Geometry: final body of the model. Coordinates: model frame, mm. Face numbers are marked on the shaded views. A direction names the side the tool comes from. Coordinates: 2 decimals unless noted, no trailing zeros. Order: outer loops, then holes, each group sorted by start corner. A loop starts at its lowest first (then second) coordinate and runs counter-clockwise, first axis right, second up. Notation, with made-up numbers: (-23, 83.5) -> (34, 83.5) arc R21 ccw to (34, 92.5) -> close; hole circle Ø3 at (49, 74.5). An arc over 180 degrees is marked (long way). Answer in a Markdown table with one row per item. Add a question column.
1) Section query B-B on x = -25. Return the cut outline in (y, z).
2) Section query D-D on y = 5. Return the cut outline in (x, z).
3) Section query C-C on y = -3. Return the cut outline in (x, z).
4) Set-up query: the marked faces 4 and 5. Return all of +Z, -Z, +X, -X, +Y, -Y with unobstructed straight access to the full face (end or side cutting, diameter ignored); none if empty.
5) Ray query, line 1 (X direction, y = 4.75, z = 0.2); line 2 (Y direction, x = 0, z = 1.85); line 3 (X direction, y = -14.25, z = 2.5). Return the intervals inside material, ascending. Write a range as from..to.
6) Section query A-A on z = 0.85. Return the cut outline in (x, y), then the cut area to 3 significant figures.
7) Contact query for flat-ended pins moving along their axis: P1, Ø6.5, axis at x = -29.75, y = 5, coming from the -Z side; P2, Ø11, axis at x = -25, y = 3, coming from the +Z side; P3, Ø3.5, axis at x = -15, y = -15.5, coming from the +Z side; P4, Ø2.5, axis at x = 0.25, y = 5, coming from the +Z side. Output: stop coordinate, or through.
8) Pull-direction query (X, two-part tool) for the marked faces 1, 2 and 3; classes: +X half, -X half, draft (parallel to the pull), parting line (faces both ways), or undercut.
```python
from build123d import *

# Parameters (mm, degrees)
EXTRUDE_1_DEPTH     = 2
EXTRUDE_2_DEPTH     = 5
EXTRUDE_3_DEPTH     = 5
SKETCH_4_R          = 2
CUT_EXTRUDE_1_DEPTH = 10
EXTRUDE_START       = -70
EXTRUDE_4_DEPTH     = 70


with BuildPart() as part:
    # 草图1 → 凸台-拉伸1 (new body)
    with BuildSketch(Plane.XY):
        Polygon((-44.754893935, 0), (15.245106065, 0), (15.245106065, -20), (20.245106065, -20), (20.245106065, 10), (15.245106065, 10), (-44.754893935, 10), (-49.754893935, 10), (-49.754893935, -20), (-44.754893935, -20), align=None)
    extrude(amount=EXTRUDE_1_DEPTH)

    # 草图2 → 凸台-拉伸2 (add)
    with BuildSketch(Plane.ZY.offset(49.754893935)):
        Polygon((0, 10), (0, -20), (2, -20), (3.461164558, -13.577882357), (3.461164558, 10), align=None)
    extrude(amount=-EXTRUDE_2_DEPTH)

    # 草图3 → 凸台-拉伸3 (add)
    with BuildSketch(Plane(origin=(20.245106065, 0, 0), x_dir=(0, 0, -1), z_dir=(1, 0, 0))):
        Polygon((-2, 10), (-3.461164558, 10), (-3.461164558, -13.577882357), (-2, -20), align=None)
    extrude(amount=-EXTRUDE_3_DEPTH)

    # 草图4 → 切除-拉伸1 (cut)
    with BuildSketch(Plane.XY.offset(2)):
        with Locations((-29.754893935, 5)):
            Circle(SKETCH_4_R)
    cut_extrude_1 = extrude(amount=-CUT_EXTRUDE_1_DEPTH, mode=Mode.SUBTRACT)

    # 镜向2: 切除-拉伸1 across plane
    add(cut_extrude_1.mirror(Plane.ZY.offset(14.754893935)), mode=Mode.SUBTRACT)

    # 草图5 → 凸台-拉伸4 (add)
    with BuildSketch(Plane.ZY.offset(49.754893935).offset(EXTRUDE_START)):
        Polygon((0, -13.225390566), (-1.541363729, -20), (0, -20), align=None)
    extrude_4 = extrude(amount=EXTRUDE_4_DEPTH)

    # 镜向3: 凸台-拉伸4 across plane
    add(extrude_4.mirror(Plane.ZY.offset(14.754893935)))


solid = part.part
```
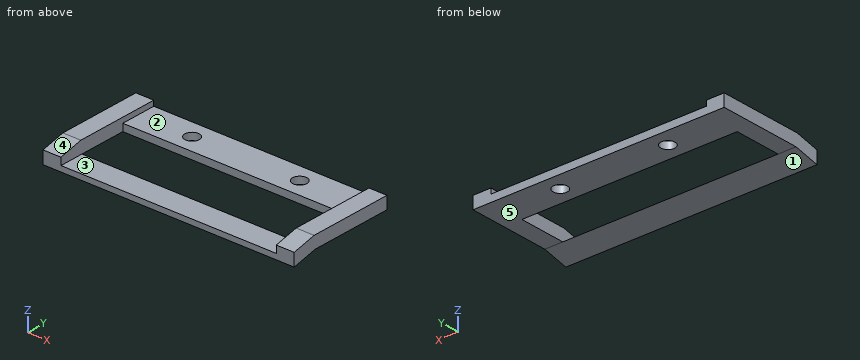
Result:
| question | item | result |
|---|---|---|
| 1 | outline | (-20, -1.54) -> (-13.23, 0) -> (-20, 0) -> close; (0, 0) -> (10, 0) -> (10, 2) -> (0, 2) -> close |
| 2 | outline | (-49.75, 0) -> (-31.75, 0) -> (-31.75, 2) -> (-44.75, 2) -> (-44.75, 3.46) -> (-49.75, 3.46) -> close; (-27.75, 0) -> (-1.75, 0) -> (-1.75, 2) -> (-27.75, 2) -> close; (2.25, 0) -> (20.25, 0) -> (20.25, 3.46) -> (15.25, 3.46) -> (15.25, 2) -> (2.25, 2) -> close |
| 3 | outline | (-49.75, 0) -> (-44.75, 0) -> (-44.75, 3.46) -> (-49.75, 3.46) -> close; (15.25, 0) -> (20.25, 0) -> (20.25, 3.46) -> (15.25, 3.46) -> close |
| 4 | face 4 | +Z, +X, -X, -Y |
| 4 | face 5 | -Z, +X, -X, +Y |
| 5 | line 1 | -49.75..-31.74, -27.77..-1.74, 2.23..20.25 |
| 5 | line 2 | 0..3.02, 6.98..10 |
| 5 | line 3 | -49.75..-44.75, 15.25..20.25 |
| 6 | outline | (-49.75, -20) -> (-44.75, -20) -> (-44.75, 0) -> (15.25, 0) -> (15.25, -20) -> (20.25, -20) -> (20.25, 10) -> (-49.75, 10) -> close; hole circle Ø4 at (-29.75, 5); hole circle Ø4 at (0.25, 5) |
| 6 | area | 875 mm2 |
| 7 | P1 | z = 0 |
| 7 | P2 | z = 2 |
| 7 | P3 | z = 0 |
| 7 | P4 | through |
| 8 | face 1 | draft |
| 8 | face 2 | undercut |
| 8 | face 3 | undercut |
